```python
from build123d import *

# Parameters (mm, degrees)
BOSS_EXTRUDE1_DEPTH   = 7.5
M6X1_0_TAPPED_HOLE1_D = 5
SKETCH6_W             = 17.945345232
SKETCH6_H             = 44.380970223
SKETCH6_R             = 2.5
BOSS_EXTRUDE2_DEPTH   = 15
CUT_EXTRUDE1_START    = -15
SKETCH8_R             = 2.5
CUT_EXTRUDE1_DEPTH    = 20


with BuildPart() as part:
    # Sketch1 → Boss-Extrude1 (new, symmetric)
    with BuildSketch(Plane(origin=(0, 0, 0), x_dir=(1, 0, 0), z_dir=(0, 1, 0))):
        with BuildLine():
            Line((-7.5, -0.193392624), (-8.972672616, 28.343633506))
            ThreePointArc((-8.972672616, 28.343633506), (0, 28.575), (8.972672616, 28.343633506))
            Line((8.972672616, 28.343633506), (7.5, -0.193392624))
            Line((7.5, -0.193392624), (7.026752085, -9.363854534))
            ThreePointArc((7.026752085, -9.363854534), (0, -16.037336717), (-7.026752085, -9.363854534))
            Line((-7.026752085, -9.363854534), (-7.5, -0.193392624))
        make_face()
    extrude(amount=BOSS_EXTRUDE1_DEPTH, both=True)

    # M6x1.0 Tapped Hole1 (through all)
    with Locations(Plane(origin=(0, 7.5, 0), x_dir=(1, 0, 0), z_dir=(0, 1, 0))):
        with Locations((0, -9.00123422), (0, 5)):
            Hole(M6X1_0_TAPPED_HOLE1_D / 2)

    # Sketch6 → Boss-Extrude2 (add, through all)
    with BuildSketch(Plane(origin=(0, 7.5, 0), x_dir=(1, 0, 0), z_dir=(0, 1, 0))):
        with Locations((0, 6.153148395)):
            Rectangle(SKETCH6_W, SKETCH6_H)
        with Locations(Location((0, -9.00123422, 0), (0, 0, 270))):
            Circle(SKETCH6_R, mode=Mode.SUBTRACT)
        with Locations(Location((0, 5, 0), (0, 0, 270))):
            Circle(SKETCH6_R, mode=Mode.SUBTRACT)
    extrude(amount=-BOSS_EXTRUDE2_DEPTH)

    # Sketch8 → Cut-Extrude1 (cut)
    with BuildSketch(Plane.XY.offset(CUT_EXTRUDE1_START)):
        Circle(SKETCH8_R)
    extrude(amount=-CUT_EXTRUDE1_DEPTH, mode=Mode.SUBTRACT)


solid = part.part
```
Here's how the part is built. I have some questions about the finished solid (model axes, mm). A direction names the side the tool comes from. Coordinates: 2 decimals unless noted, no trailing zeros. Write each loop counter-clockwise with the first axis right and the second up, starting at its lowest first coordinate (ties: lowest second). Pieces come first, ordered by that corner, then holes. Notation, with made-up numbers: (70, 5.25) -> (77, 5.25) arc R16 ccw to (77, 10.25) -> close; hole circle Ø8 at (42.25, 37). An arc over 180 degrees is marked (long way). Use a Markdown table: item, result. Add a question column.
(1) If we section it at B-B, the plane z = -5: Write out the boundary of the cut face in (x, y).
(2) I'm going to push flat-ended pins straight in: P1, Ø2, axis at x = 1, y = -4.5, coming from the -Z side (3 decimals); P2, Ø2.5, axis at x = 0, y = 1, coming from the -Z side. Where does each tip first touch, or does it pass through?
(3) If we section it at C-C, the plane z = -24: Write out the boundary of the cut face in (x, y).
(4) Please list where these lines run through material, in increasing order: line 1 (Z direction, x = 0, y = 0.75); line 2 (Y direction, x = 0, z = -17.75); line 3 (Z direction, x = 1, y = 2).
(5) For faces 1 (the flat face through (8.973, 0, -6)), 2 (the flat face through (0, 0, -15)), which set-ups out of +Z, -Z, +X, -X, +Y, -Y let a thin tool reach every point of the face, with its end or its side?
(6) We'd pull the mould along Y, two halves only. Please class faces 3 (the flat face through (-2, -7.5, -7)), 4 (the cylindrical face through (-0.54, -2.44, -21.69)), 5 (the flat face through (0, 0, 16.037)), 6 (the flat face through (-2, 7.5, -7)): +Y half, -Y half, draft (parallel to the pull), parting line (faces both ways), or undercut.
(7) If we section it at A-A, the plane x = 0: Write out the boundary of the cut face in (y, z) (3 decimals).
(8) If we section it at D-D, the plane y = 2: Write out the boundary of the cut face in (x, z), and give its area (3 significant figures).
Outcome:
| question | item | result |
|---|---|---|
| 1 | outline | (-8.97, -7.5) -> (-2.5, -7.5) -> (-2.5, 7.5) -> (-8.97, 7.5) -> close; (2.5, -7.5) -> (8.97, -7.5) -> (8.97, 7.5) -> (2.5, 7.5) -> close |
| 2 | P1 | stops at z = -28.575 |
| 2 | P2 | stops at z = -15 |
| 3 | outline | (-8.97, -7.5) -> (8.97, -7.5) -> (8.97, 7.5) -> (-8.97, 7.5) -> close; hole circle Ø5 at (0, 0) |
| 4 | line 1 | z = -15 to -7.5, -2.5 to 6.5, 11.5 to 16.04 |
| 4 | line 2 | y = -7.5 to -2.5, 2.5 to 7.5 |
| 4 | line 3 | z = -15 to -7.29, -2.71 to 6.71, 11.29 to 16.04 |
| 5 | face 1 | +Z, -Z, +X, +Y, -Y |
| 5 | face 2 | -Z |
| 6 | face 3 | -Y half |
| 6 | face 4 | undercut |
| 6 | face 5 | draft |
| 6 | face 6 | +Y half |
| 7 | outline | (-7.5, -28.575) -> (-2.5, -28.575) -> (-2.5, -15) -> (2.5, -15) -> (2.5, -28.575) -> (7.5, -28.575) -> (7.5, -7.5) -> (-7.5, -7.5) -> close; (-7.5, -2.5) -> (7.5, -2.5) -> (7.5, 6.501) -> (-7.5, 6.501) -> close; (-7.5, 11.501) -> (7.5, 11.501) -> (7.5, 16.037) -> (-7.5, 16.037) -> close |
| 8 | outline | (-8.97, -28.34) arc R174.1 ccw to (-1.5, -28.57) -> (-1.5, -15) -> (1.5, -15) -> (1.5, -28.57) arc R174.1 ccw to (8.97, -28.34) -> (8.97, 16.04) -> (-8.97, 16.04) -> close; hole circle Ø5 at (0, -5); hole circle Ø5 at (0, 9) |
| 8 | area | 719 mm^2 |
